from build123d import *

# Parameters (mm, degrees)
ESQUISSE1_W        = 440
ESQUISSE1_H        = 360
ESQUISSE1_R        = 2.7
BOSS_EXTRU_1_DEPTH = 5
CONG_1_R           = 40


with BuildPart() as part:
    # Esquisse1 → Boss.-Extru.1 (new body)
    with BuildSketch(Plane(origin=(0, 0, 0), x_dir=(1, 0, 0), z_dir=(0, 1, 0))):
        with Locations((220, 180)):
            Rectangle(ESQUISSE1_W, ESQUISSE1_H)
        with Locations((40, 350)):
            Circle(ESQUISSE1_R, mode=Mode.SUBTRACT)
        with Locations((130, 350)):
            Circle(ESQUISSE1_R, mode=Mode.SUBTRACT)
        with Locations((220, 350)):
            Circle(ESQUISSE1_R, mode=Mode.SUBTRACT)
        with Locations((310, 350)):
            Circle(ESQUISSE1_R, mode=Mode.SUBTRACT)
        with Locations((400, 350)):
            Circle(ESQUISSE1_R, mode=Mode.SUBTRACT)
        with Locations((400, 10)):
            Circle(ESQUISSE1_R, mode=Mode.SUBTRACT)
        with Locations((310, 10)):
            Circle(ESQUISSE1_R, mode=Mode.SUBTRACT)
        with Locations((220, 10)):
            Circle(ESQUISSE1_R, mode=Mode.SUBTRACT)
        with Locations((130, 10)):
            Circle(ESQUISSE1_R, mode=Mode.SUBTRACT)
        with Locations((40, 10)):
            Circle(ESQUISSE1_R, mode=Mode.SUBTRACT)
        with Locations((10, 217.36725867)):
            Circle(ESQUISSE1_R, mode=Mode.SUBTRACT)
        with Locations((10, 317.36725867)):
            Circle(ESQUISSE1_R, mode=Mode.SUBTRACT)
        with Locations((10, 42.63274133)):
            Circle(ESQUISSE1_R, mode=Mode.SUBTRACT)
        with Locations((10, 142.63274133)):
            Circle(ESQUISSE1_R, mode=Mode.SUBTRACT)
        with Locations((430, 142.63274133)):
            Circle(ESQUISSE1_R, mode=Mode.SUBTRACT)
        with Locations((430, 42.63274133)):
            Circle(ESQUISSE1_R, mode=Mode.SUBTRACT)
        with Locations((430, 317.36725867)):
            Circle(ESQUISSE1_R, mode=Mode.SUBTRACT)
        with Locations((430, 217.36725867)):
            Circle(ESQUISSE1_R, mode=Mode.SUBTRACT)
        with BuildLine():
            Line((370, 250), (420, 250))
            Line((420, 250), (420, 110))
            Line((420, 110), (370, 110))
            ThreePointArc((370, 110), (300, 180), (370, 250))
        make_face(mode=Mode.SUBTRACT)
    extrude(amount=BOSS_EXTRU_1_DEPTH)

    # Congé1
    cong_1_edges = [part.edges().sort_by_distance(p)[0] for p in [
        (420, 2.5, -110),
        (420, 2.5, -250),
    ]]
    fillet(cong_1_edges, radius=CONG_1_R)


solid = part.part
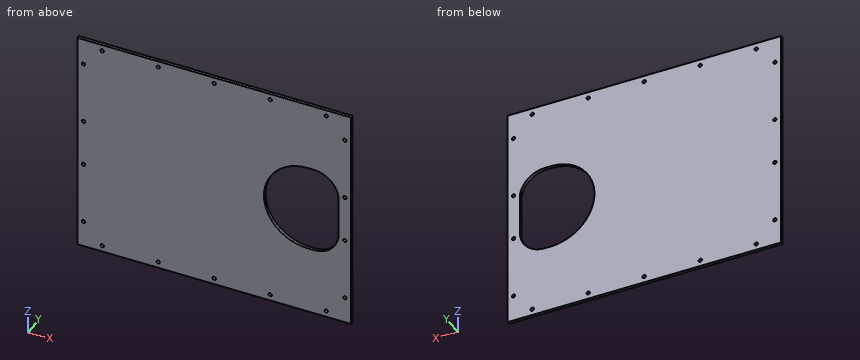
Geometry: final body of the model. Coordinates: model frame, mm. Give positions to 0.01 mm unless a question says otherwise; leave off trailing zeros. Order: outer loops, then holes, each group sorted by start corner. A loop starts at its lowest first (then second) coordinate and runs counter-clockwise, first axis right, second up. Notation, with made-up numbers: (70, 86) -> (113, 86) arc R25 ccw to (113, 118) -> close; hole circle Ø9 at (15, 22). An arc over 180 degrees is marked (long way). Put each result on its own line as item: value.
Q1. Section A-A, the plane z = -180. Return loops of the section in (x, y), then the cut area to 3 significant figures.
Here are the results:
outline: (0, 0) -> (300, 0) -> (300, 5) -> (0, 5) -> close; (420, 0) -> (440, 0) -> (440, 5) -> (420, 5) -> close
area: 1,600 mm^2
Q2. Pin query (flat end, axial travel): pin 1 (5 mm diameter, centred on x = 430, z = -142.63, fed in from -Y). Return the tip coordinate at first contact, or that it passes through.
Here are the results:
pin 1: passes through
Q3. Section B-B, the plane x = 319.5. Return loops of the section in (y, z), then the cut area to 3 significant figures.
Here are the results:
outline: (0, -360) -> (5, -360) -> (5, -228.47) -> (0, -228.47) -> close; (0, -131.53) -> (5, -131.53) -> (5, 0) -> (0, 0) -> close
area: 1,320 mm^2
Q4. Material intervals for L1, parallel to Z at x = 130, y = 3.9; L2, parallel to X at y = 1.35, z = -350; L3, parallel to Z at x = 10, y = 3.6, sorted ascending.
Here are the results:
L1: z = -360 to -352.7, -347.3 to -12.7, -7.3 to 0
L2: x = 0 to 37.3, 42.7 to 127.3, 132.7 to 217.3, 222.7 to 307.3, 312.7 to 397.3, 402.7 to 440
L3: z = -360 to -320.07, -314.67 to -220.07, -214.67 to -145.33, -139.93 to -45.33, -39.93 to 0
Q5. Section C-C, the plane y = 4. Count the separate pieces of the cut face and the enclosed holes in it, then the cut area to 3 significant figures.
Here are the results:
separate pieces: 1
enclosed holes: 19
area: 144,000 mm^2
